Source: CAD feature listing. Evaluate the final solid. Frame: model axes, mm. A direction names the side the tool comes from. Give positions to 0.01 mm unless a question says otherwise; leave off trailing zeros. Loops run counter-clockwise (first coordinate to the right, second up) from the corner with the lowest first, then second, coordinate; pieces in that order, holes last. Notation, with made-up numbers: M 20,-29.75 L 34,-29.75 A32 ccw 34,-3.75 Z; hole C -20.5,-29.75 d8. An arc over 180 degrees is marked long. Put each result on its own line as item: value. Start each with the question number.
```python
from build123d import *

# Parameters (mm, degrees)
SKETCH1_W           = 108
SKETCH1_H           = 76.2
BOSS_EXTRUDE1_DEPTH = 101.6
SKETCH2_R           = 71.616075106
BOSS_EXTRUDE2_DEPTH = 203.2
SKETCH4_R           = 71.616075106
BOSS_EXTRUDE3_DEPTH = 350
BOSS_EXTRUDE3_DRAFT = -8


# Read off the part's stored shape, not the designer's step: Shell1
with BuildPart() as part:
    # Sketch1 → Boss-Extrude1 (new body)
    with BuildSketch(Plane(origin=(0, 0, 0), x_dir=(1, 0, 0), z_dir=(0, 1, 0))):
        Rectangle(SKETCH1_W, SKETCH1_H)
    extrude(amount=BOSS_EXTRUDE1_DEPTH)

    # Sketch2 → Boss-Extrude2 (add)
    with BuildSketch(Plane(origin=(0, 101.6, 0), x_dir=(1, 0, 0), z_dir=(0, 1, 0))):
        with Locations(Location((0, 0, 0), (0, 0, 270))):
            Circle(SKETCH2_R)
    extrude(amount=BOSS_EXTRUDE2_DEPTH)


with BuildPart() as boss_extrude3_tool:
    # Sketch4 → Boss-Extrude3 (with draft: the straight prism first)
    with BuildSketch(Plane(origin=(0, 304.8, 0), x_dir=(1, 0, 0), z_dir=(0, 1, 0))):
        with Locations(Location((0, 0, 0), (0, 0, 270))):
            Circle(SKETCH4_R)
    extrude(amount=BOSS_EXTRUDE3_DEPTH)
    # Boss-Extrude3: the draft: its side faces are tilted about the plane it starts from
    boss_extrude3_sides = [boss_extrude3_tool.faces().sort_by_distance(p)[0] for p in [
        (0, 479.8, -71.616075106),
    ]]
    draft(boss_extrude3_sides, Plane(origin=(0, 304.8, 0), x_dir=(1, 0, 0), z_dir=(0, 1, 0)), BOSS_EXTRUDE3_DRAFT)


with BuildPart() as part_1:
    add(part.part)

    # Boss-Extrude3: add boss_extrude3_tool
    add(boss_extrude3_tool.part)

    # Shell1 outline → Shell1 (revolve, cut)
    with BuildSketch(Plane.XY):
        Polygon((0, 654.8), (0, 139.7), (33.516075106, 139.7), (33.516075106, 307.464211535), (82.330936739, 654.8), align=None)
    revolve(axis=Axis((0, 0, 0), (0, 1, 0)), mode=Mode.SUBTRACT)


solid = part_1.part
```
1. Section D-D, the plane y = 496.5. Output: boundary loops of the cut face in (x, z), plus the area to 3 significant figures.
2. Section B-B, the plane x = 0. Output: boundary loops of the cut face in (y, z), plus the area to 3 significant figures.
3. Ray query, line 1 (X direction, y = 250, z = 0); line 2 (Y direction, x = -17.5, z = 16); line 3 (Z direction, x = -22, y = 378). Return the intervals inside material, ascending.
4. Section C-C, the plane y = 235. Output: boundary loops of the cut face in (x, z).
5. Contact query for flat-ended pins moving along their axis: pin 1 (12 mm diameter, centred on y = 315, z = 60, fed in from -X); pin 2 (1.5 mm diameter, centred on x = 18, y = 451, fed in from +Z); pin 3 (6 mm diameter, centred on y = 436.5, z = 79.5, fed in from -X). Output: stop coordinate, or through.
6. Pull-direction query (X, two-part tool) for faces 4 (the face through (-54, 50, 1)), 5 (the face through (-1, 50, -38.1)), 6 (the face through (-4.36, 224.76, -33.23)), 7 (the face through (55.575, 483.563, -17.501)); classes: released by +X, released by -X, zero draft, split by the parting line, or undercut.
7. Set-up query: faces 1 (the face through (71.007, 201.778, -9.323)), 2 (the face through (54, 50, 1)), 3 (the face through (0, 139.7, 0)). Return all of +Z, -Z, +X, -X, +Y, -Y with unobstructed straight access to the full face (end or side cutting, diameter ignored); none if empty.
8. Section A-A, the plane z = 0. Output: boundary loops of the cut face in (x, y), plus the area to 3 significant figures.
Results found:
1. outline: C 0,0 d197.12; hole C 0,0 d120.17
1. area: 19,200 mm²
2. outline: M 0,-38.1 L 101.6,-38.1 L 101.6,-71.62 L 304.8,-71.62 L 654.8,-120.81 L 654.8,-82.33 L 307.46,-33.52 L 139.7,-33.52 L 139.7,33.52 L 307.46,33.52 L 654.8,82.33 L 654.8,120.81 L 304.8,71.62 L 101.6,71.62 L 101.6,38.1 L 0,38.1 Z
2. area: 52,700 mm²
3. line 1: -71.62 to -33.52, 33.52 to 71.62
3. line 2: 0 to 139.7
3. line 3: -78.89 to -37.44, 37.44 to 78.89
4. outline: C 0,0 d143.23; hole C 0,0 d67.03
5. pin 1: x = -49.31
5. pin 2: z = 90.57
5. pin 3: x = -47.71
6. face 4: released by -X
6. face 5: zero draft
6. face 6: undercut
6. face 7: undercut
7. face 1: -Y
7. face 2: +Z, -Z, +X, -Y
7. face 3: +Y
8. outline: M -120.81,654.8 L -71.62,304.8 L -71.62,101.6 L -54,101.6 L -54,0 L 54,0 L 54,101.6 L 71.62,101.6 L 71.62,304.8 L 120.81,654.8 L 82.33,654.8 L 33.52,307.46 L 33.52,139.7 L -33.52,139.7 L -33.52,307.46 L -82.33,654.8 Z
8. area: 55,900 mm²
